The figure shows three views and two pictorial views of one solid part (mm, origin at its lowest corner). Answer the questions. A direction names the side the tool comes from. Round coordinates to 2 decimals unless told otherwise and drop trailing zeros. Order: outer loops, then holes, each group sorted by start corner. A loop starts at its lowest first (then second) coordinate and runs counter-clockwise, first axis right, second up. Notation, with made-up numbers: (8.25, 33.25) -> (53.25, 33.25) arc R27 ccw to (53.25, 57.25) -> close; hole circle Ø10 at (34.25, -21). An arc over 180 degrees is marked (long way). One line per item, written item: value. Start each with the question number.
1. Flat-ended cylindrical pins translate along their axes: pin 1 Ø8 at (x, y) = (17.5, 17) entering from +Z; pin 2 Ø1.5 at (x, z) = (8, 24.5) entering from +Y; pin 3 Ø1.8 at (x, y) = (18, 46.5) entering from +Z; pin 4 Ø2.5 at (x, y) = (16.5, 38.5) entering from +Z. Find the tip coordinate at first contact, or state that the pin passes through.
2. Section D-D (x = 18) is taken. Give the vertices of the cut face in (y, z), then the cut area to 3 significant figures.
3. Consider line 1 (Y direction, x = 18, z = 2.1); line 2 (Y direction, x = 4, z = 16.25); line 3 (Y direction, x = 4, z = 9.95). Determine where each line is inside the solid, lowest interval first.
4. Section A-A (y = 22.5) is taken. Give the vertices of the cut face in (x, z), then the cut area to 3 significant figures.
5. Section C-C (z = 17.25) is taken. Give the vertices of the cut face in (x, y), then the cut area to 3 significant figures.
6. For the marked faces 4, 5, 6 and 7, determine the directions among +Z, -Z, +X, -X, +Y, -Y from which every point of the face is accessible in a straight line to the end or side of a thin tool.
7. The mould has two halves that part along Y. Classify the marked faces 1, 2 and 3: released by +Y, released by -Y, zero draft, split by the parting line, or undercut.
8. Section B-B (x = 4) is taken. Give the vertices of the cut face in (y, z), then the cut area to 3 significant figures.
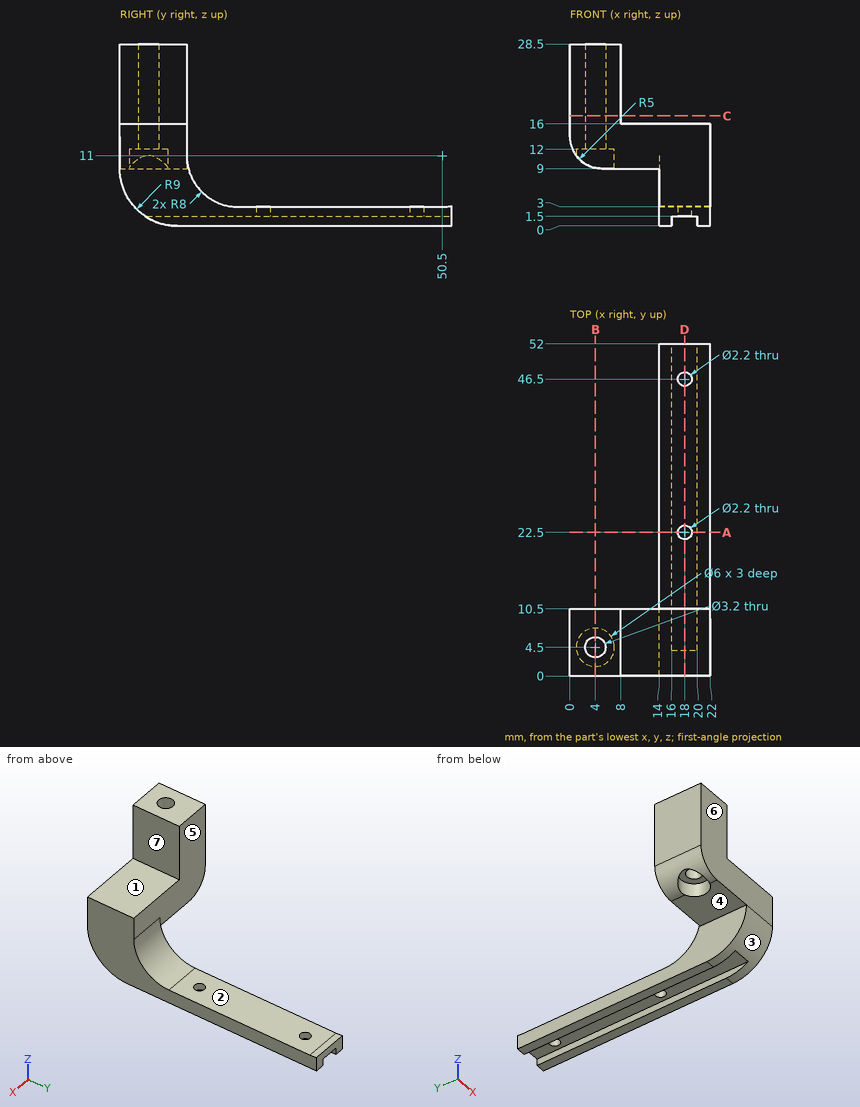
Answer:
1. pin 1: z = 5.19
1. pin 2: y = 10.5
1. pin 3: through
1. pin 4: z = 3
2. outline: (0, 9) arc R9 ccw to (4.03, 1.5) -> (21.4, 1.5) -> (21.4, 3) -> (18.5, 3) arc R8 cw to (10.5, 11) -> (10.5, 16) -> (0, 16) -> close; (23.6, 1.5) -> (45.4, 1.5) -> (45.4, 3) -> (23.6, 3) -> close; (47.6, 1.5) -> (52, 1.5) -> (52, 3.14) arc R8 cw to (50.5, 3) -> (47.6, 3) -> close
2. area: 213 mm^2
3. line 1: 3.22 to 21.4, 23.6 to 45.4, 47.6 to 52
3. line 2: 0 to 2.9, 6.1 to 10.5
3. line 3: 0 to 1.5, 7.5 to 10.5
4. outline: (14, 0) -> (16, 0) -> (16, 1.5) -> (16.9, 1.5) -> (16.9, 3) -> (14, 3) -> close; (19.1, 1.5) -> (20, 1.5) -> (20, 0) -> (22, 0) -> (22, 3) -> (19.1, 3) -> close
4. area: 14.7 mm^2
5. outline: (0, 0) -> (8, 0) -> (8, 10.5) -> (0, 10.5) -> close; hole circle Ø3.2 at (4, 4.5)
5. area: 76.0 mm^2
6. face 4: -Z, -X, +Y, -Y
6. face 5: +Z, -X, +Y
6. face 6: +Z, -Z, +X, -X, -Y
6. face 7: +Z, +X, +Y, -Y
7. face 1: zero draft
7. face 2: undercut
7. face 3: released by -Y
8. outline: (0, 9.1) -> (1.5, 9.1) -> (1.5, 12) -> (2.9, 12) -> (2.9, 28.5) -> (0, 28.5) -> close; (6.1, 12) -> (7.5, 12) -> (7.5, 9.1) -> (10.5, 9.1) -> (10.5, 28.5) -> (6.1, 28.5) -> close
8. area: 133 mm^2
